```python
from build123d import *

# Parameters (mm, degrees)
F0_R     = 2
F1_DEPTH = 3


with BuildPart() as f1:
    # F0 (on Front) → F1 (new body)
    with BuildSketch(Plane.XZ):
        with BuildLine():
            Line((-154.777424, 73.567189), (-158.777424, 73.567189))
            ThreePointArc((-158.777424, 73.567189), (-145.59723, 41.747384), (-113.777424, 28.567189))
            Line((-113.777424, 28.567189), (-13.777424, 28.567189))
            ThreePointArc((-13.777424, 28.567189), (18.042381, 41.747384), (31.222576, 73.567189))
            Line((31.222576, 73.567189), (27.222576, 73.567189))
            ThreePointArc((27.222576, 73.567189), (18.79852, 48.671249), (-3.011954, 34.005786))
            ThreePointArc((-3.011954, 34.005786), (-6.66184, 34.41013), (-9.05112, 37.198768))
            ThreePointArc((-9.05112, 37.198768), (-14.104804, 40.55646), (-18.676404, 36.567189))
            ThreePointArc((-18.676404, 36.567189), (-20.413106, 33.694206), (-23.575383, 32.567189))
            Line((-23.575383, 32.567189), (-103.979465, 32.567189))
            ThreePointArc((-103.979465, 32.567189), (-107.141743, 33.694206), (-108.878445, 36.567189))
            ThreePointArc((-108.878445, 36.567189), (-113.450045, 40.55646), (-118.503728, 37.198768))
            ThreePointArc((-118.503728, 37.198768), (-120.893009, 34.41013), (-124.542895, 34.005786))
            ThreePointArc((-124.542895, 34.005786), (-146.353369, 48.671249), (-154.777424, 73.567189))
        make_face()
        with Locations((-113.777424, 35.567189)):
            Circle(F0_R, mode=Mode.SUBTRACT)
        with Locations((-13.777424, 35.567189)):
            Circle(F0_R, mode=Mode.SUBTRACT)
    extrude(amount=F1_DEPTH)


solid = f1.part
```
CAD build for the part. Positions are in the model's coordinates, mm. A direction names the side the tool comes from. Round coordinates to 2 decimals unless told otherwise and drop trailing zeros. Loops run counter-clockwise (first coordinate to the right, second up) from the corner with the lowest first, then second, coordinate; pieces in that order, holes last. Notation, with made-up numbers: M 3,15 L 19,15 A24 cw 19,31 Z; hole C -18.75,46.25 d4. An arc over 180 degrees is marked long. Use a Markdown table: item, result. Add a question column.
(1) Cut at B-B (y = -0.9). Give the cut face in (x, z), and give its area (3 significant figures).
(2) Drill centre lines: line 1 (X direction, y = -2.45, z = 39.5); line 2 (X direction, y = -2.35, z = 38.5); line 3 (Z direction, x = -27, y = -0.25). Where is each one in solid material? Low to high.
(3) Which spindle directions (+Z, -Z, +X, -X, +Y, -Y) get a long thin tool onto all of the face, cutting with end or side? Do faces 4 (the face through (-64, -1, 28.567)), 5 (the face through (-63, -1, 32.567)). Say none if no direction does.
(4) Cut at D-D (z = 69.5). Give the cut face in (x, y), and give its area (3 significant figures).
(5) Cut at C-C (x = -93). Give the cut face in (y, z), and give its area (3 significant figures).
(6) Cut at A-A (z = 45). Give the cut face in (x, y), and give its area (3 significant figures).
(7) Flat gauge pins, fed straight in: pin 1 (5 mm diameter, centred on x = -13.78, z = 35.57, fed in from -Y); pin 2 (1.5 mm diameter, centred on x = -126.5, y = -2, fed in from -Z); pin 3 (1 mm diameter, centred on y = -2, z = 62, fed in from +X). Where does each tip first touch, or does it go through?
(8) Pull direction Z, two halves, no side cores. Call faces 1 (the face through (17.69, -1.48, 41.4)), 2 (the face through (-14.04, -1.48, 37.55)), 3 (the face through (-146.12, -1.48, 48.37)): +Z half, -Z half, draft (parallel to the pull), parting line (faces both ways), or undercut.
Geometry says:
| question | item | result |
|---|---|---|
| 1 | outline | M -158.78,73.57 A45 ccw -113.78,28.57 L -13.78,28.57 A45 ccw 31.22,73.57 L 27.22,73.57 A41 cw -3.01,34.01 A5 cw -9.05,37.2 A5 ccw -18.68,36.57 A5 cw -23.58,32.57 L -103.98,32.57 A5 cw -108.88,36.57 A5 ccw -118.5,37.2 A5 cw -124.54,34.01 A41 cw -154.78,73.57 Z; hole C -113.78,35.57 d4; hole C -13.78,35.57 d4 |
| 1 | area | 1,070 mm² |
| 2 | line 1 | x = -143.18 to -136.59, -116.86 to -110.69, -16.86 to -10.69, 9.04 to 15.62 |
| 2 | line 2 | x = -141.98 to -135.02, -117.83 to -109.73, -17.83 to -9.73, 7.47 to 14.42 |
| 2 | line 3 | z = 28.57 to 32.57 |
| 3 | face 4 | -Z, +X, -X, +Y, -Y |
| 3 | face 5 | +Z, +Y, -Y |
| 4 | outline | M -158.59,-3 L -154.58,-3 L -154.58,0 L -158.59,0 Z; M 27.02,-3 L 31.04,-3 L 31.04,0 L 27.02,0 Z |
| 4 | area | 24.1 mm² |
| 5 | outline | M -3,28.57 L 0,28.57 L 0,32.57 L -3,32.57 Z |
| 5 | area | 12.0 mm² |
| 6 | outline | M -148.55,-3 L -143.19,-3 L -143.19,0 L -148.55,0 Z; M 15.63,-3 L 20.99,-3 L 20.99,0 L 15.63,0 Z |
| 6 | area | 32.2 mm² |
| 7 | pin 1 | stops at y = -3 |
| 7 | pin 2 | stops at z = 30.19 |
| 7 | pin 3 | stops at x = 29.84 |
| 8 | face 1 | -Z half |
| 8 | face 2 | undercut |
| 8 | face 3 | +Z half |
